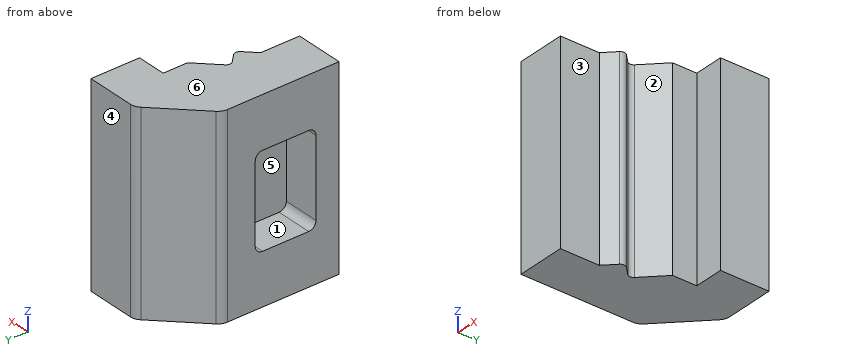
from build123d import *

# Parameters (mm, degrees)
F0_W     = 10
F0_H     = 10
F1_DEPTH = 80
F2_R     = 2
F3_R     = 2
F4_SIZE  = 20
F5_W     = 25
F5_H     = 38
F6_DEPTH = 15
F7_R     = 3
F8_R     = 5


with BuildPart() as f1:
    # F0 (on Top) → F1 (new body)
    with BuildSketch(Plane.XY):
        Polygon((-57.7475710213, 35.1921368795), (-57.7475710213, 15.1921368795), (-37.7475710213, 15.1921368795), (-27.7475710213, 15.1921368795), (-15.7475710213, 15.1921368795), (-15.7475710213, 35.1921368795), align=None)
        Polygon((-37.7475710213, 15.1921368795), (-57.7475710213, 15.1921368795), (-57.7475710213, -32.8078631205), (-37.7475710213, -32.8078631205), (-37.7475710213, -16.8078631205), (-37.7475710213, -4.8078631205), (-37.7475710213, 5.1921368795), align=None)
        with Locations((-32.7475710213, 10.1921368795)):
            Rectangle(F0_W, F0_H)
        Polygon((-27.7475710213, 5.1921368795), (-37.7475710213, 5.1921368795), (-37.7475710213, -4.8078631205), align=None)
        Polygon((-31.7475710213, -10.8078631205), (-37.7475710213, -4.8078631205), (-37.7475710213, -16.8078631205), align=None)
    extrude(amount=F1_DEPTH)

    # F2
    f2_edges = [f1.edges().sort_by_distance(p)[0] for p in [
        (-31.747571, -10.807863, 40),
    ]]
    fillet(f2_edges, radius=F2_R)

    # F3
    f3_edges = [f1.edges().sort_by_distance(p)[0] for p in [
        (-37.747571, -4.807863, 40),
    ]]
    fillet(f3_edges, radius=F3_R)

    # F4
    f4_edges = [f1.edges().sort_by_distance(p)[0] for p in [
        (-57.747571, 35.192137, 40),
    ]]
    chamfer(f4_edges, length=F4_SIZE)

    # F5 (on face) → F6 (cut)
    with BuildSketch(Plane(origin=(-57.7475710213, 0, 0), x_dir=(0, -1, 0), z_dir=(-1, 0, 0))):
        with Locations((10.8078631205, 40)):
            Rectangle(F5_W, F5_H)
    extrude(amount=-F6_DEPTH, mode=Mode.SUBTRACT)

    # F7
    f7_edges = [f1.edges().sort_by_distance(p)[0] for p in [
        (-50.247571, 1.692137, 21),
        (-50.247571, 1.692137, 59),
        (-50.247571, -23.307863, 59),
        (-50.247571, -23.307863, 21),
    ]]
    fillet(f7_edges, radius=F7_R)

    # F8
    f8_edges = [f1.edges().sort_by_distance(p)[0] for p in [
        (-37.747571, 35.192137, 40),
        (-57.747571, 15.192137, 40),
    ]]
    fillet(f8_edges, radius=F8_R)


solid = f1.part
Design review of the part built by this model. Coordinates are the model's own, in mm. Face numbers are marked on the shaded views. A direction names the side the tool comes from. Round coordinates to 2 decimals unless told otherwise and drop trailing zeros. Write each loop counter-clockwise with the first axis right and the second up, starting at its lowest first coordinate (ties: lowest second). Pieces come first, ordered by that corner, then holes. Notation, with made-up numbers: M 5.5,-19.5 L 49.5,-19.5 A30 ccw 49.5,19.5 Z; hole C 71,40 d6. An arc over 180 degrees is marked long. One line per item, written item: value. Start each with the question number.
1. For the marked faces 1, 2 and 3, list the 3-axis set-ups (+Z, -Z, +X, -X, +Y, -Y) from which the entire face can be reached by the end or side of a thin tool; tool diameter is ignored.
2. Draft analysis for pull direction Z (two halves, no side actions). For the marked faces 4, 5 and 6, state which applies: pulls with the +Z half, pulls with the -Z half, needs draft (parallel to the pull), parting line crosses it, or undercut.
3. To check wall thickness, follow probe 1 along Z at (x, y) = (-47.5, -17.5); probe 2 along X at (y, z) = (7, 8); probe 3 along Y at (x, z) = (-21.5, 48). State the ranges of each line that lie inside material, in increasing order. Write a range as from..to.
4. Clearance check with flat-ended pins moving along their axes: P1, Ø8, axis at y = 9, z = 37.5, coming from the +X side; P2, Ø16.5, axis at x = -53, z = 43, coming from the +Y side; P3, Ø17.5, axis at y = -28.5, z = 23, coming from the +X side; P4, Ø10, axis at x = -43.5, y = 12.5, coming from the -Z side. State where each tip first meets the part, or that it passes through.
5. Take a section at A-A on z = 19.5. State the section outline as (x, y) points.
6. Take a section at C-C on y = -11. State the section outline as (x, z) points, then the cut area to 3 significant figures.
7. Take a section at D-D on x = -19.5. State the section outline as (y, z) points.
8. Take a section at B-B on x = -50.5. State the section outline as (y, z) points, then the cut area to 3 significant figures.
Computed:
1. face 1: -X
1. face 2: +Z, -Z, +X
1. face 3: +Z, -Z, +X, -Y
2. face 4: needs draft
2. face 5: undercut
2. face 6: pulls with the +Z half
3. probe 1: z = 0..21, 59..80
3. probe 2: x = -57.75..-27.75
3. probe 3: y = 15.19..35.19
4. P1: stops at x = -27.75
4. P2: stops at y = 28.19
4. P3: stops at x = -37.75
4. P4: stops at z = 0
5. outline: M -57.75,-32.81 L -37.75,-32.81 L -37.75,-16.81 L -33.16,-12.22 A2 ccw -33.16,-9.39 L -36.33,-6.22 A2 cw -36.33,-3.39 L -27.75,5.19 L -27.75,15.19 L -15.75,15.19 L -15.75,35.19 L -35.68,35.19 A5 ccw -39.21,33.73 L -56.28,16.66 A5 ccw -57.75,13.12 Z
6. outline: M -57.75,0 L -32.59,0 L -32.59,80 L -57.75,80 L -57.75,59 L -42.75,59 L -42.75,21 L -57.75,21 Z
6. area: 1,440 mm²
7. outline: M 15.19,0 L 35.19,0 L 35.19,80 L 15.19,80 Z
8. outline: M -32.81,0 L 22.44,0 L 22.44,80 L -32.81,80 Z; hole M -23.31,24 A3 ccw -20.31,21 L -1.31,21 A3 ccw 1.69,24 L 1.69,56 A3 ccw -1.31,59 L -20.31,59 A3 ccw -23.31,56 Z
8. area: 3,480 mm²
